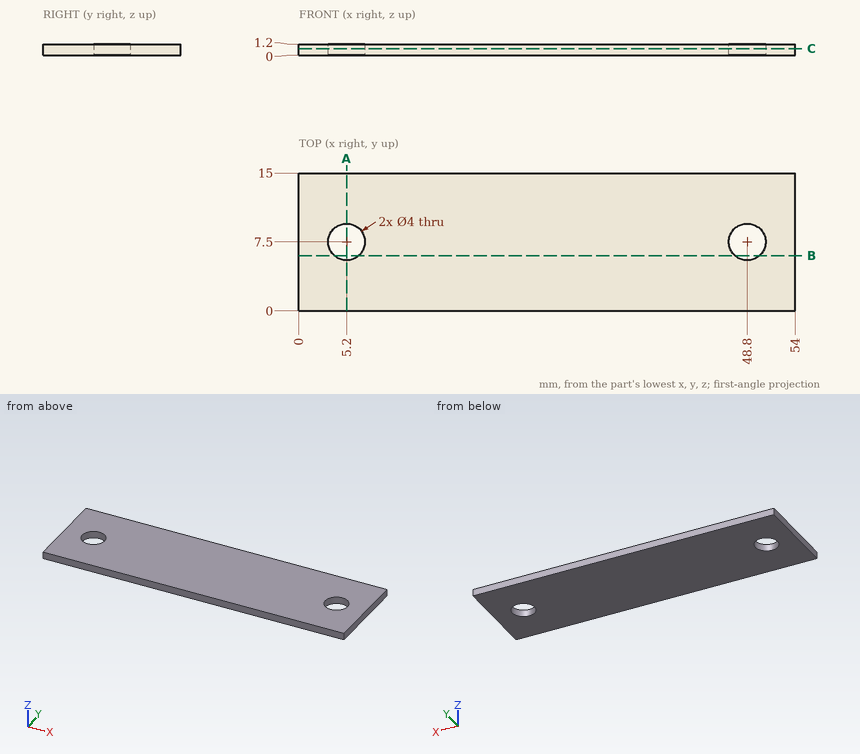
Verification items for this drawing (mm, ordinates from the low corner). Give positions to 0.01 mm unless a question says otherwise; leave off trailing zeros. Loops run counter-clockwise (first coordinate to the right, second up) from the corner with the lowest first, then second, coordinate; pieces in that order, holes last. Notation, with made-up numbers: M 2,-32.5 L 29,-32.5 A22 ccw 29,-14.5 Z; hole C -32,54 d1. An arc over 180 degrees is marked long. Answer as a JSON object with one key per item and string values. Group by question number.
Item 1: Sectioned sample at B-B on y = 6. Record the boundary of the cut face in (x, z), plus the area to 3 significant figures.
Item 2: Sectioned sample at C-C on z = 0.7. Record the boundary of the cut face in (x, y).
Item 3: Sectioned sample at A-A on x = 5.2. Record the boundary of the cut face in (y, z), plus the area to 3 significant figures.
Item 4: Material ranges on L1, parallel to Y at x = 48.8, z = 0.6; L2, parallel to X at y = 8.5, z = 0.85; L3, parallel to X at y = 7, z = 0.4, recorded low to high.
Findings below:
{
 "1": {"outline": "M 0,0 L 3.88,0 L 3.88,1.2 L 0,1.2 Z; M 6.52,0 L 47.48,0 L 47.48,1.2 L 6.52,1.2 Z; M 50.12,0 L 54,0 L 54,1.2 L 50.12,1.2 Z", "area": "58.5 mm2"},
 "2": {"outline": "M 0,0 L 54,0 L 54,15 L 0,15 Z; hole C 5.2,7.5 d4; hole C 48.8,7.5 d4"},
 "3": {"outline": "M 0,0 L 5.5,0 L 5.5,1.2 L 0,1.2 Z; M 9.5,0 L 15,0 L 15,1.2 L 9.5,1.2 Z", "area": "13.2 mm2"},
 "4": {"L1": "0 to 5.5, 9.5 to 15", "L2": "0 to 3.47, 6.93 to 47.07, 50.53 to 54", "L3": "0 to 3.26, 7.14 to 46.86, 50.74 to 54"}
}
